Check sheet for the modelled part. Datum: model origin and axes. Units: mm. A direction names the side the tool comes from. Coordinates: 2 decimals unless noted, no trailing zeros. Use CSV: the item, a comma, the result in double quotes. Start each with the question number.
1. Set-up check for faces 4 (the face through (11, -5, 4.762)), 5 (the face through (4.762, 12, 1)), 6 (the face through (-7.31, 18.27, 8.05)): record each of +Z, -Z, +X, -X, +Y, -Y from which the full face is reachable in a straight line by a thin tool's end or side.
2. Release check for a two-part mould opening along Y. For faces 1 (the face through (-18.4, 17.463, 14.7)), 2 (the face through (11, -17.462, 2)), 3 (the face through (-19.833, -4.296, 12.528)) record: pulls with the +Y half, pulls with the -Y half, needs draft (parallel to the pull), parting line crosses it, or undercut.
3. Thickness scan on L1, parallel to X at y = -6.5, z = 6; L2, parallel to Y at x = -17.5, z = 8.5; L3, parallel to Y at x = -18, z = 9.25. Record the ranges inside material, lowest first.
4. Gauge pin test, flat ends, axial feed: pin 1 (1.9 mm diameter, centred on y = -3, z = 14, fed in from +X); pin 2 (1.9 mm diameter, centred on x = -2, z = 11, fed in from -Y); pin 3 (0.8 mm diameter, centred on x = 18, y = -7.5, fed in from +Z) (3 decimals). Record the tip position at first contact, or that the pin passes through.
5. Sectioned sample at A-A, the plane x = 12.5. Count the separate pieces of the cut face and the enclosed holes in it, and give its area (3 significant figures).
```python
from build123d import *

# Parameters (mm, degrees)
F0_W      = 38.1
F0_H      = 38.1
F1_DEPTH  = 15.875
F2_W      = 12.7
F2_H      = 34.925
F3_DEPTH  = 11.1125
F4_W      = 11.1125
F4_H      = 12.7
F5_DEPTH  = 38.101
F6_W      = 23.8125
F6_H      = 11.1125
F7_DEPTH  = 1.5875
F8_W      = 7.9375
F8_H      = 3.175
F8_H_2    = 3.96875
F9_DEPTH  = 4.7625
F11_DEPTH = 1.5875
F12_R     = 1.190625
F13_DEPTH = 9.525
F14_R     = 1.190625
F15_DEPTH = 9.525
F16_W     = 12.7
F16_H     = 20.6375
F17_DEPTH = 3.96875
F18_W     = 14.2875
F18_H     = 6.35
F19_DEPTH = 25.4
F20_R     = 1.5875
F21_DEPTH = 2.38125
F22_R     = 0.79375


with BuildPart() as f1:
    # F0 (on Top) → F1 (new body)
    with BuildSketch(Plane.XY):
        Rectangle(F0_W, F0_H)
    extrude(amount=F1_DEPTH)

    # F2 (on face) → F3 (cut)
    with BuildSketch(Plane.XY.offset(15.875)):
        with Locations((11.1125, 0)):
            Rectangle(F2_W, F2_H)
    extrude(amount=-F3_DEPTH, mode=Mode.SUBTRACT)

    # F4 (on face) → F5 (cut, through all)
    with BuildSketch(Plane.YZ.offset(19.05)):
        with Locations((11.90625, 7.9375)):
            Rectangle(F4_W, F4_H)
    extrude(amount=-F5_DEPTH, mode=Mode.SUBTRACT)

    # F6 (on face) → F7 (cut, through all)
    with BuildSketch(Plane(origin=(0, 0, 0), x_dir=(1, 0, 0), z_dir=(0, 0, -1))):
        with Locations((-7.14375, -11.90625)):
            Rectangle(F6_W, F6_H)
    extrude(amount=-F7_DEPTH, mode=Mode.SUBTRACT)

    # F8 (on face) → F9 (cut, through all)
    with BuildSketch(Plane.XY.offset(4.7625)):
        with Locations((11.1125, 0.79375)):
            Rectangle(F8_W, F8_H)
        with Locations((11.1125, -13.096875)):
            Rectangle(F8_W, F8_H_2)
    extrude(amount=-F9_DEPTH, mode=Mode.SUBTRACT)

    # F10 (on face) → F11 (cut)
    with BuildSketch(Plane(origin=(0, 19.05, 0), x_dir=(-1, 0, 0), z_dir=(0, 1, 0))):
        Polygon((19.05, 0), (19.05, 15.875), (-4.7625, 0), align=None)
    extrude(amount=-F11_DEPTH, mode=Mode.SUBTRACT)

    # F12 (on face) → F13 (join)
    with BuildSketch(Plane(origin=(-19.05, 0, 0), x_dir=(0, -1, 0), z_dir=(-1, 0, 0))):
        with BuildLine():
            Line((-6.35, 5.55625), (-6.35, 11.90625))
            Line((-6.35, 11.90625), (-7.14375, 11.90625))
            ThreePointArc((-7.14375, 11.90625), (-10.31875, 8.73125), (-7.14375, 5.55625))
            Line((-7.14375, 5.55625), (-6.35, 5.55625))
        make_face()
        with Locations((-7.9375, 8.73125)):
            Circle(F12_R, mode=Mode.SUBTRACT)
    extrude(amount=-F13_DEPTH)

    # F14 (on face) → F15 (join)
    with BuildSketch(Plane(origin=(-19.05, 0, 0), x_dir=(0, -1, 0), z_dir=(-1, 0, 0))):
        with BuildLine():
            Line((20.6375, 11.90625), (19.05, 11.90625))
            Line((19.05, 11.90625), (19.05, 5.55625))
            Line((19.05, 5.55625), (20.6375, 5.55625))
            ThreePointArc((20.6375, 5.55625), (23.8125, 8.73125), (20.6375, 11.90625))
        make_face()
        with Locations((20.6375, 8.73125)):
            Circle(F14_R, mode=Mode.SUBTRACT)
    extrude(amount=-F15_DEPTH)

    # F16 (on face) → F17 (cut)
    with BuildSketch(Plane(origin=(0, 0, 0), x_dir=(1, 0, 0), z_dir=(0, 0, -1))):
        with Locations((11.1125, 7.14375)):
            Rectangle(F16_W, F16_H)
    extrude(amount=-F17_DEPTH, mode=Mode.SUBTRACT)

    # F18 (on face) → F19 (cut)
    with BuildSketch(Plane.YZ.offset(19.05)):
        with Locations((-3.96875, 12.7)):
            Rectangle(F18_W, F18_H)
    extrude(amount=-F19_DEPTH, mode=Mode.SUBTRACT)

    # F20 (on face) → F21 (join)
    with BuildSketch(Plane(origin=(-19.05, 0, 0), x_dir=(0, -1, 0), z_dir=(-1, 0, 0))):
        with Locations((5.55625, 13.49375)):
            Circle(F20_R)
        with Locations((5.55625, 3.96875)):
            Circle(F20_R)
    extrude(amount=F21_DEPTH)

    # F22
    f22_edges = [f1.edges().sort_by_distance(p)[0] for p in [
        (-21.43125, -3.96875, 13.49375),
        (-21.43125, -3.96875, 3.96875),
    ]]
    fillet(f22_edges, radius=F22_R)


solid = f1.part
```
Completed:
1,face 4,"+Z"
1,face 5,"-Z, -X"
1,face 6,"-Z, -X, +Y"
2,face 1,"pulls with the +Y half"
2,face 2,"undercut"
2,face 3,"parting line crosses it"
3,L1,"-19.05 to 4.76, 17.46 to 19.05"
3,L2,"-23.8 to -21.81, -19.47 to 6.77, 9.11 to 10.31"
3,L3,"-23.77 to -21.71, -19.57 to 6.87, 9.01 to 10.28"
4,pin 1,"x = -6.35"
4,pin 2,"y = -19.05"
4,pin 3,"z = 9.525"
5,separate pieces,"3"
5,enclosed holes,"0"
5,area,"93.9 mm²"
